Input: part model. Units: mm. Frame: model coordinates. Round coordinates to 2 decimals unless told otherwise and drop trailing zeros. Write each loop counter-clockwise with the first axis right and the second up, starting at its lowest first coordinate (ties: lowest second). Pieces come first, ordered by that corner, then holes. Notation, with made-up numbers: (-4.5, 19) - (31.5, 19) arc R8 ccw to (31.5, 28) - close; hole circle Ø11 at (51.25, -25). An arc over 180 degrees is marked (long way). Use one line per item in the form item = value.
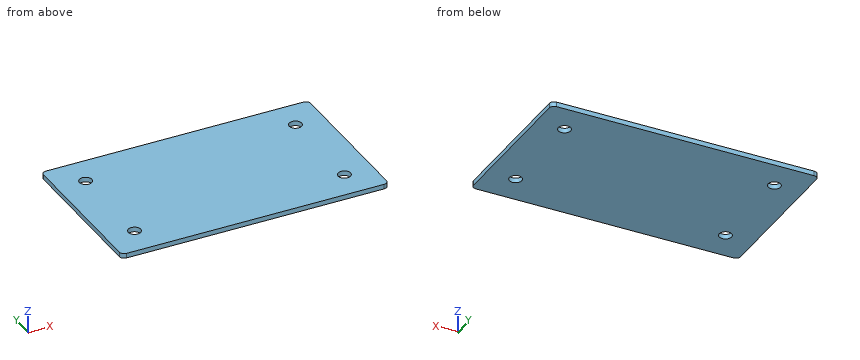
```python
from build123d import *

# Parameters (mm, degrees)
SKETCH_1_W          = 280
SKETCH_1_H          = 165
EXTRUDE_1_DEPTH     = 5
SKETCH_2_R          = 6.5
CUT_EXTRUDE_1_DEPTH = 6
FILLET_1_R          = 5


with BuildPart() as part:
    # 草图1 → 凸台-拉伸1 (new body)
    with BuildSketch(Plane.XY):
        Rectangle(SKETCH_1_W, SKETCH_1_H)
    extrude(amount=EXTRUDE_1_DEPTH)

    # 草图2 → 切除-拉伸1 (cut)
    with BuildSketch(Plane.XY.offset(5)):
        with Locations((-110, 50)):
            Circle(SKETCH_2_R)
        with Locations((110, 50)):
            Circle(SKETCH_2_R)
        with Locations((-110, -50)):
            Circle(SKETCH_2_R)
        with Locations((110, -50)):
            Circle(SKETCH_2_R)
    extrude(amount=-CUT_EXTRUDE_1_DEPTH, mode=Mode.SUBTRACT)

    # 圆角1
    fillet_1_edges = [part.edges().sort_by_distance(p)[0] for p in [
        (140, -82.5, 2.5),
        (-140, -82.5, 2.5),
        (-140, 82.5, 2.5),
        (140, 82.5, 2.5),
    ]]
    fillet(fillet_1_edges, radius=FILLET_1_R)


solid = part.part
```
(1) Cut plane B-B on x = 110. Output: boundary loops of the cut face in (y, z).
Derived:
outline = (-82.5, 0) - (-56.5, 0) - (-56.5, 5) - (-82.5, 5) - close; (-43.5, 0) - (43.5, 0) - (43.5, 5) - (-43.5, 5) - close; (56.5, 0) - (82.5, 0) - (82.5, 5) - (56.5, 5) - close
(2) Material intervals for L1, parallel to Y at x = 110, z = 2.05; L2, parallel to Y at x = 108, z = 1.45, sorted ascending.
Derived:
L1 = -82.5 to -56.5, -43.5 to 43.5, 56.5 to 82.5
L2 = -82.5 to -56.18, -43.82 to 43.82, 56.18 to 82.5
(3) Cut plane A-A on y = 50. Output: boundary loops of the cut face in (x, z), then the cut area to 3 significant figures.
Derived:
outline = (-140, 0) - (-116.5, 0) - (-116.5, 5) - (-140, 5) - close; (-103.5, 0) - (103.5, 0) - (103.5, 5) - (-103.5, 5) - close; (116.5, 0) - (140, 0) - (140, 5) - (116.5, 5) - close
area = 1,270 mm^2
